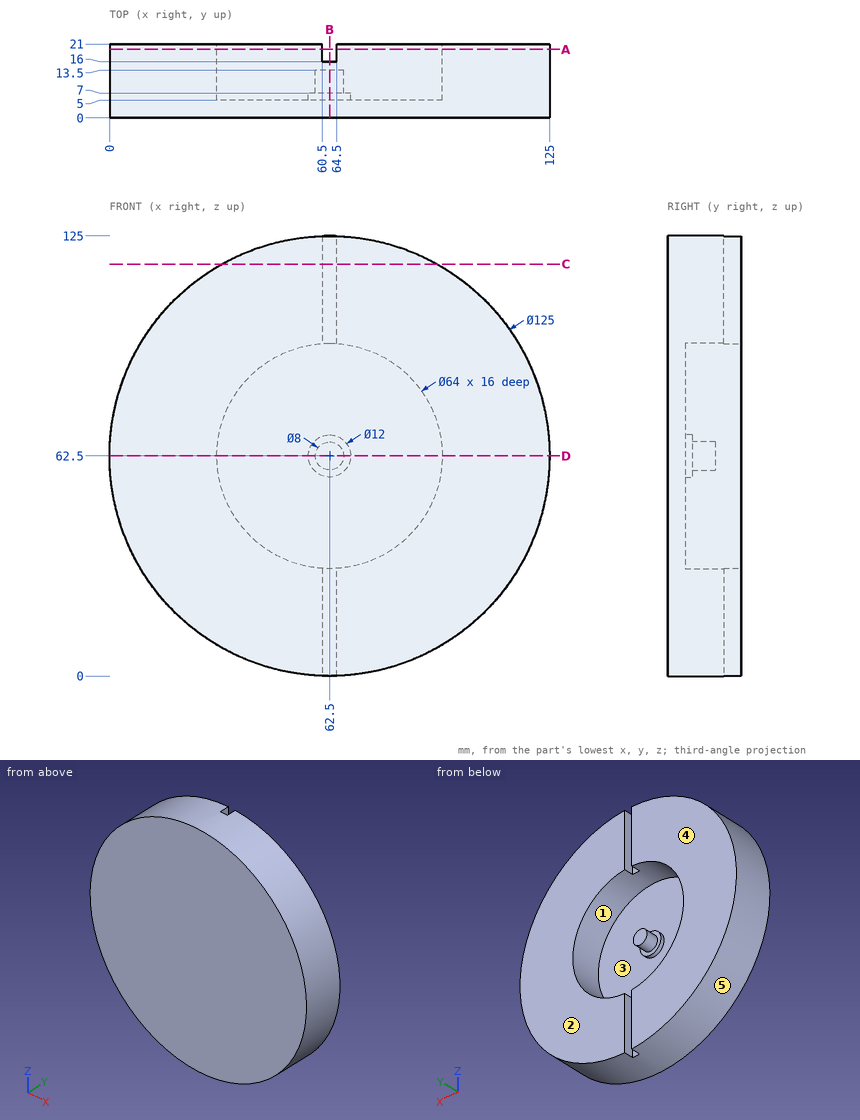
Input: dimensioned drawing with shaded views. Units: mm. Origin: part minimum x, y, z. A direction names the side the tool comes from. Give positions to 0.01 mm unless a question says otherwise; leave off trailing zeros. Order: outer loops, then holes, each group sorted by start corner. A loop starts at its lowest first (then second) coordinate and runs counter-clockwise, first axis right, second up. Notation, with made-up numbers: (-6, 75.5) -> (52, 75.5) arc R20 cw to (52, 89.5) -> close; hole circle Ø8 at (-14, 47.5). An arc over 180 degrees is marked (long way). Use one line per item in the form item = value.
1) Reachability of the marked faces 1 and 2 from +Z, -Z, +X, -X, +Y, -Y: full face, straight path, thin tool, end or side. Return the list, or none.
Response values:
face_1 = +Y
face_2 = +Z, -Z, +X, -X, +Y
2) Line query: probe 1 along X at (y, z) = (12, 62.5); probe 2 along Y at (x, z) = (61.5, 79.5); probe 3 along X at (y, z) = (9.5, 49). Output: solid intervals per line, ascending.
Response values:
probe_1 = 0 to 30.5, 58.5 to 66.5, 94.5 to 125
probe_2 = 0 to 5
probe_3 = 1.48 to 33.49, 91.51 to 123.52
3) Section A-A, the plane y = 19.5. Return loops of the section in (x, z), and give its area (3 significant figures).
Response values:
outline = (60.5, 0.03) -> (60.5, 30.56) arc R32 cw to (60.5, 94.44) -> (60.5, 124.97) arc R62.5 ccw to start; (64.5, 0.03) arc R62.5 ccw to (64.5, 124.97) -> (64.5, 94.44) arc R32 cw to (64.5, 30.56) -> close
area = 8,810 mm^2
4) First-contact query: pin 1 Ø8 at (x, z) = (54, 61.5) entering from +Y; pin 2 Ø2.5 at (y, z) = (17.5, 103.5) entering from +X; pin 3 Ø1.2 at (x, z) = (63.5, 102.5) entering from +Y. Flat tips, straight axial feed; report the tip coordinate or a pass-through.
Response values:
pin_1 = 7
pin_2 = 110.73
pin_3 = 16
5) Section C-C, the plane z = 117. Return loops of the section in (x, y), and give its area (3 significant figures).
Response values:
outline = (31.91, 0) -> (93.09, 0) -> (93.09, 21) -> (64.5, 21) -> (64.5, 16) -> (60.5, 16) -> (60.5, 21) -> (31.91, 21) -> close
area = 1,260 mm^2
6) Section B-B, the plane x = 62.5. Return loops of the section in (y, z), and give its area (3 significant figures).
Response values:
outline = (0, 0) -> (16, 0) -> (16, 30.5) -> (5, 30.5) -> (5, 56.5) -> (7, 56.5) -> (7, 58.5) -> (13.5, 58.5) -> (13.5, 66.5) -> (7, 66.5) -> (7, 68.5) -> (5, 68.5) -> (5, 94.5) -> (16, 94.5) -> (16, 125) -> (0, 125) -> close
area = 1,370 mm^2
7) Section D-D, the plane z = 62.5. Return loops of the section in (x, y).
Response values:
outline = (0, 0) -> (125, 0) -> (125, 21) -> (94.5, 21) -> (94.5, 5) -> (68.5, 5) -> (68.5, 7) -> (66.5, 7) -> (66.5, 13.5) -> (58.5, 13.5) -> (58.5, 7) -> (56.5, 7) -> (56.5, 5) -> (30.5, 5) -> (30.5, 21) -> (0, 21) -> close
8) Mould query, pull axis X, two halves, no side actions, for the marked faces 3, 4 and 5. Classes: pulls with the +X half, pulls with the -X half, needs draft (parallel to the pull), parting line crosses it, or undercut.
Response values:
face_3 = undercut
face_4 = needs draft
face_5 = parting line crosses it
